from build123d import *

# Parameters (mm, degrees)
PAD_DEPTH       = 1.5
SKETCH002_W     = 9.788774
SKETCH002_H     = 1.27
POCKET001_DEPTH = 0.635
SKETCH001_W     = 9.785776
SKETCH001_H     = 0.5
POCKET_DEPTH    = 0.5


with BuildPart() as part:
    # Sketch → Pad (new body)
    with BuildSketch(Plane.XY):
        Polygon((-12.5, 6), (-5, 6), (-5, 0), (5, 0), (5, 6), (12.5, 6), (12.5, -4), (-12.5, -4), align=None)
    extrude(amount=-PAD_DEPTH)

    # Sketch002 → Pocket001 (cut)
    with BuildSketch(Plane.XY):
        with Locations((8.541229, 4.25644)):
            Rectangle(SKETCH002_W, SKETCH002_H)
        with Locations((8.541229, 1.71644)):
            Rectangle(SKETCH002_W, SKETCH002_H)
    extrude(amount=-POCKET001_DEPTH, mode=Mode.SUBTRACT)

    # Sketch001 → Pocket (cut)
    with BuildSketch(Plane.XY):
        with Locations((-8.271684, 4.25644)):
            Rectangle(SKETCH001_W, SKETCH001_H)
        with Locations((-8.271684, 1.71644)):
            Rectangle(SKETCH001_W, SKETCH001_H)
    extrude(amount=-POCKET_DEPTH, mode=Mode.SUBTRACT)


solid = part.part
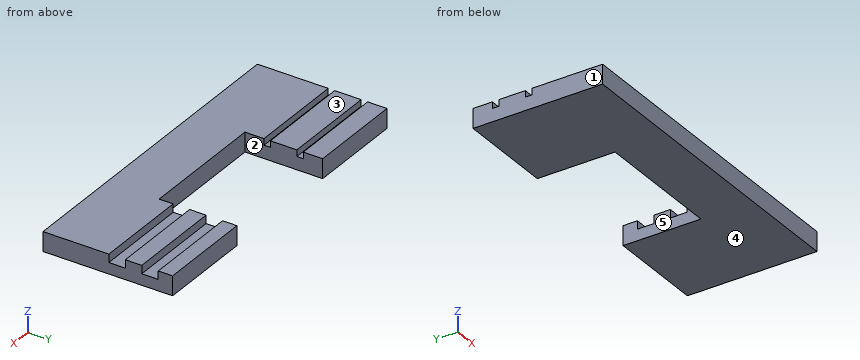
Input: part model. Units: mm. Frame: model coordinates. Face numbers are marked on the shaded views. A direction names the side the tool comes from. Coordinates: 2 decimals unless noted, no trailing zeros. Loops run counter-clockwise (first coordinate to the right, second up) from the corner with the lowest first, then second, coordinate; pieces in that order, holes last. Notation, with made-up numbers: (-4.75, 11) -> (3.25, 11) arc R28 cw to (3.25, 50) -> close; hole circle Ø10 at (20.25, -31.75). An arc over 180 degrees is marked (long way). One line per item, written item: value.
(1) Cut plane B-B (z = -1.05). Output: boundary loops of the cut face in (x, y), then the cut area to 3 significant figures.
Answer below:
outline: (-12.5, -4) -> (12.5, -4) -> (12.5, 6) -> (5, 6) -> (5, 0) -> (-5, 0) -> (-5, 6) -> (-12.5, 6) -> close
area: 190 mm2
(2) Cut plane A-A (x = -7). Output: boundary loops of the cut face in (y, z).
Answer below:
outline: (-4, -1.5) -> (6, -1.5) -> (6, 0) -> (4.51, 0) -> (4.51, -0.5) -> (4.01, -0.5) -> (4.01, 0) -> (1.97, 0) -> (1.97, -0.5) -> (1.47, -0.5) -> (1.47, 0) -> (-4, 0) -> close
(3) Draft query along X for the marked faces 1, 2 and 3. Return one class per face: pulls with the +X half, pulls with the -X half, needs draft (parallel to the pull), parting line crosses it, or undercut.
Answer below:
face 1: pulls with the -X half
face 2: undercut
face 3: needs draft
(4) Pin query (flat end, axial travel): pin 1 Ø0.8 at (x, z) = (-1.5, -0.5) entering from +Y. Return the tip coordinate at first contact, or that it passes through.
Answer below:
pin 1: stops at y = 0
(5) Cut plane C-C (y = 0.75). Output: boundary loops of the cut face in (x, z), then the cut area to 3 significant figures.
Answer below:
outline: (-12.5, -1.5) -> (-5, -1.5) -> (-5, 0) -> (-12.5, 0) -> close; (5, -1.5) -> (12.5, -1.5) -> (12.5, 0) -> (5, 0) -> close
area: 22.5 mm2
(6) Ray query, line 1 along Y through (x, z) = (-6.25, -0.4); line 2 along X through (y, z) = (3.75, -0.95); line 3 along Y through (x, z) = (-4.25, -0.3). Return the intervals inside material, ascending.
Answer below:
line 1: y = -4 to 1.47, 1.97 to 4.01, 4.51 to 6
line 2: x = -12.5 to -5, 5 to 12.5
line 3: y = -4 to 0
(7) Cut plane D-D (x = -3.25). Output: boundary loops of the cut face in (y, z), then the cut area to 3 significant figures.
Answer below:
outline: (-4, -1.5) -> (0, -1.5) -> (0, 0) -> (-4, 0) -> close
area: 6.00 mm2
(8) Set-up query: the marked faces 4 and 5. Return all of +Z, -Z, +X, -X, +Y, -Y with unobstructed straight access to the full face (end or side cutting, diameter ignored); none if empty.
Answer below:
face 4: -Z, +X, -X, +Y, -Y
face 5: +Z, -Z, +Y
